For this review, take the finished solid that the model builds, in its own axes (mm). Face numbers are marked on the shaded views. A direction names the side the tool comes from. Coordinates: 2 decimals unless noted, no trailing zeros. Order: outer loops, then holes, each group sorted by start corner. A loop starts at its lowest first (then second) coordinate and runs counter-clockwise, first axis right, second up. Notation, with made-up numbers: (-22.75, 62.25) -> (-2.75, 62.25) arc R23 ccw to (-2.75, 92.25) -> close; hole circle Ø8 at (1.25, -22). An arc over 180 degrees is marked (long way). Answer as a JSON object with one key per item and string values. Group by question number.
1) Wall thickness on L1, parallel to Y at x = 25, z = 4.25; L2, parallel to X at y = -21.5, z = 1; L3, parallel to X at y = 9, z = 3: over which ranges is each line inside the solid? List them lowest first.
2) For pin 1 (0.8 mm diameter, centred on x = 29, z = 7.5, fed in from -Y); pin 2 (3 mm diameter, centred on x = 42.5, y = 0, fed in from +Z); pin 3 (0.8 mm diameter, centred on x = 27.5, z = 7.5, fed in from +Y), all flat-tipped, find the tip position at first contact; note any pin that passes through.
3) Machinability: for the marked faces 1 and 2, which of the approach directions +Z, -Z, +X, -X, +Y, -Y give a long, thin tool a straight path to every point of the face, cutting with its end or side? Answer none if there is none.
4) Draft analysis for pull direction Y (two halves, no side actions). For the marked faces 3, 4 and 5, state which applies: +Y half, -Y half, draft (parallel to the pull), parting line (faces both ways), or undercut.
5) Add section C-C, the plane x = 29. Write out the cut boundary in (y, z), then the cut area to 3 significant figures.
6) Add section A-A, the plane y = 0. Write out the cut boundary in (x, z).
7) Add section B-B, the plane x = 0. Count the separate pieces of the cut face and the enclosed holes in it, then the cut area to 3 significant figures.
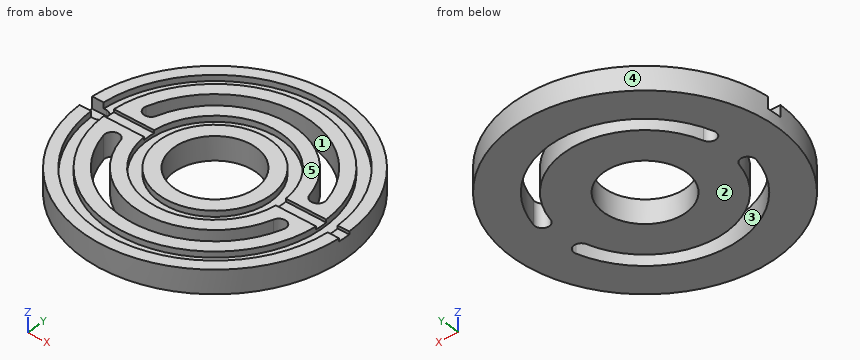
from build123d import *

# Parameters (mm, degrees)
SKETCH_1_R            = 45
EXTRUDE_1_DEPTH       = 8
SKETCH_2_R            = 14
CUT_EXTRUDE_1_DEPTH   = 65.140470843
SKETCH_3_R            = 41
SKETCH_3_R_2          = 37
CUT_EXTRUDE_1_2_DEPTH = 2
CUT_EXTRUDE_2_DEPTH   = 4
CUT_EXTRUDE_3_DEPTH   = 65.140470843
SKETCH_6_R            = 23
SKETCH_6_R_2          = 19
CUT_EXTRUDE_2_2_DEPTH = 2
SKETCH_7_W            = 18
SKETCH_7_H            = 4
SKETCH_7_W_2          = 26
CUT_EXTRUDE_3_2_DEPTH = 1


with BuildPart() as part:
    # 草图1 → 凸台-拉伸1 (new body)
    with BuildSketch(Plane.XY):
        Circle(SKETCH_1_R)
    extrude(amount=EXTRUDE_1_DEPTH)

    # 草图2 → Cut-Extrude 1 (cut, through all)
    with BuildSketch(Plane.XY.offset(8)):
        Circle(SKETCH_2_R)
    extrude(amount=-CUT_EXTRUDE_1_DEPTH, mode=Mode.SUBTRACT)

    # 草图3 → Cut-Extrude 1 2 (cut)
    with BuildSketch(Plane.XY.offset(8)):
        Circle(SKETCH_3_R)
        Circle(SKETCH_3_R_2, mode=Mode.SUBTRACT)
    extrude(amount=-CUT_EXTRUDE_1_2_DEPTH, mode=Mode.SUBTRACT)

    # 草图4 → Cut-Extrude 2 (cut)
    with BuildSketch(Plane.XY.offset(8)):
        with BuildLine():
            Line((-45, 2.5), (-40, 2.5))
            ThreePointArc((-40, 2.5), (-37.5, 0), (-40, -2.5))
            Line((-40, -2.5), (-45, -2.5))
            ThreePointArc((-45, -2.5), (-47.5, 0), (-45, 2.5))
        make_face()
    extrude(amount=-CUT_EXTRUDE_2_DEPTH, mode=Mode.SUBTRACT)

    # 草图5 → Cut-Extrude 3 (cut, through all)
    with BuildSketch(Plane.XY.offset(8)):
        with BuildLine():
            ThreePointArc((31.392589354, 8.411618966), (0, 32.5), (-31.392589354, 8.411618966))
            ThreePointArc((-31.392589354, 8.411618966), (-29.624822401, 5.349756787), (-26.562960223, 7.11752374))
            ThreePointArc((-26.562960223, 7.11752374), (0, 27.5), (26.562960223, 7.11752374))
            ThreePointArc((26.562960223, 7.11752374), (29.624822401, 5.349756787), (31.392589354, 8.411618966))
        make_face()
    cut_extrude_3 = extrude(amount=-CUT_EXTRUDE_3_DEPTH, mode=Mode.SUBTRACT)

    # 镜向1: Cut-Extrude 3 across plane
    add(cut_extrude_3.mirror(Plane.ZX), mode=Mode.SUBTRACT)

    # 草图6 → Cut-Extrude 2 2 (cut)
    with BuildSketch(Plane.XY.offset(8)):
        Circle(SKETCH_6_R)
        Circle(SKETCH_6_R_2, mode=Mode.SUBTRACT)
    extrude(amount=-CUT_EXTRUDE_2_2_DEPTH, mode=Mode.SUBTRACT)

    # 草图7 → Cut-Extrude 3 2 (cut)
    with BuildSketch(Plane.XY.offset(8)):
        with Locations((-28, 0)):
            Rectangle(SKETCH_7_W, SKETCH_7_H)
        with Locations((32, 0)):
            Rectangle(SKETCH_7_W_2, SKETCH_7_H)
    extrude(amount=-CUT_EXTRUDE_3_2_DEPTH, mode=Mode.SUBTRACT)


solid = part.part
Output values:
{
 "1": {"L1": "y = -37.42 to -20.77, -11.46 to 11.46, 20.77 to 37.42", "L2": "x = -39.53 to -24.37, -17.15 to 17.15, 24.37 to 39.53", "L3": "x = -44.09 to -31.23, -25.99 to -10.72, 10.72 to 25.99, 31.23 to 44.09"},
 "2": {"pin 1": "stops at y = -34.74", "pin 2": "stops at z = 7", "pin 3": "stops at y = 35.92"},
 "3": {"face 1": "+Z, -Z", "face 2": "-Z, +X, -X, +Y, -Y"},
 "4": {"face 3": "undercut", "face 4": "parting line", "face 5": "draft"},
 "5": {"outline": "(-34.41, 0) -> (-14.67, 0) -> (-14.67, 8) -> (-22.98, 8) -> (-22.98, 6) -> (-28.98, 6) -> (-28.98, 8) -> (-34.41, 8) -> close; (-5.26, 0) -> (5.26, 0) -> (5.26, 8) -> (2, 8) -> (2, 7) -> (-2, 7) -> (-2, 8) -> (-5.26, 8) -> close; (14.67, 0) -> (34.41, 0) -> (34.41, 8) -> (28.98, 8) -> (28.98, 6) -> (22.98, 6) -> (22.98, 8) -> (14.67, 8) -> close", "area": "372 mm²"},
 "6": {"outline": "(-45, 0) -> (-14, 0) -> (-14, 8) -> (-19, 8) -> (-19, 6) -> (-23, 6) -> (-23, 7) -> (-37, 7) -> (-37, 6) -> (-37.5, 6) -> (-37.5, 4) -> (-45, 4) -> close; (14, 0) -> (45, 0) -> (45, 7) -> (41, 7) -> (41, 6) -> (37, 6) -> (37, 7) -> (23, 7) -> (23, 6) -> (19, 6) -> (19, 8) -> (14, 8) -> close"},
 "7": {"separate pieces": "4", "enclosed holes": "0", "area": "384 mm²"}
}
